Design review of the part built by this model. Coordinates are the model's own, in mm. A direction names the side the tool comes from. Coordinates: 2 decimals unless noted, no trailing zeros. Loops run counter-clockwise (first coordinate to the right, second up) from the corner with the lowest first, then second, coordinate; pieces in that order, holes last. Notation, with made-up numbers: (50, 74.25) - (92, 74.25) arc R19 ccw to (92, 92.25) - close; hole circle Ø2 at (6.5, 54). An arc over 180 degrees is marked (long way). Use one line per item in the form item = value. Start each with the question number.
(1) Clearance check with flat-ended pins moving along their axes: pin 1 Ø12 at (x, y) = (564, -11) entering from +Z; pin 2 Ø10 at (x, z) = (315.5, 11) entering from -Y; pin 3 Ø1.5 at (x, y) = (233.5, 1) entering from -Z; pin 4 Ø8 at (x, y) = (186.5, -3) entering from +Z. State where each tip first meets the part, or that it passes through.
(2) For L1, parallel to Z at x = 85, y = -23.5; L2, parallel to X at y = -25.5, z = 33.5; L3, parallel to Z at x = 700, y = 4, list the stretches that pass through material, from the lowest coordinate up.
(3) Add section B-B (x = 85). State the section outline as (y, z) points, plus the area to 3 significant figures.
(4) Add section C-C (z = -53). State the section outline as (x, y) points, plus the area to 3 significant figures.
(5) Tool access review of faces 1 (the face through (235.18, -9.86, 30.56)), 2 (the face through (396, -5, 1)), 3 (the face through (189.012, -16.504, -30.269)): name each direction out of +Z, -Z, +X, -X, +Y, -Y from which nothing blocks a thin tool from reaching the whole face with its end or side.
(6) The part is to be moulded in two halves that separate along X. For faces 4 (the face through (439.49, -3.5, -21.13)), 5 (the face through (685, -32.5, -17)), 6 (the face through (54.399, -9.86, -63.033)), say which applies: pulls with the +X half, pulls with the -X half, needs draft (parallel to the pull), parting line crosses it, or undercut.
(7) Add section A-A (y = 6). State the section outline as (x, z) points, plus the area to 3 significant figures.
```python
from build123d import *

# Parameters (mm, degrees)
F0_R          = 29
F1_DEPTH      = 20
F3_DEPTH      = 5
F5_DEPTH      = 5
F6_R          = 4.99999
F7_R          = 4.99999
F8_R          = 29
F8_R_2        = 22.5
F8_R_3        = 24
F9_DEPTH      = 12.5
F9_DEPTH_BACK = 32.5


# Not quite as in the source:
# - a fillet or chamfer is up to 0.001 mm smaller than in the source, because OpenCascade refuses the exact size


with BuildPart() as f1:
    # F0 (on Front) → F1 (new body)
    with BuildSketch(Plane.XZ):
        with BuildLine():
            Line((228.5028561992, 32.1062064806), (97.7975828549, 74.4774856478))
            ThreePointArc((97.7975828549, 74.4774856478), (54.8450921386, 63.5119541924), (46.3006134969, 20.0130895684))
            ThreePointArc((46.3006134969, 20.0130895684), (48.3193625322, 12.9155090118), (49, 5.5678746945))
            Line((49, 5.5678746945), (49, -5.5678746945))
            ThreePointArc((49, -5.5678746945), (48.3193625322, -12.9155090118), (46.3006134969, -20.0130895684))
            ThreePointArc((46.3006134969, -20.0130895684), (54.8450921386, -63.5119541924), (97.7975828549, -74.4774856478))
            Line((97.7975828549, -74.4774856478), (228.5028561992, -32.1062064806))
            ThreePointArc((228.5028561992, -32.1062064806), (235.0832865864, -30.5729005697), (241.8279137151, -30.1690491218))
            Line((241.8279137151, -30.1690491218), (698.9728356822, -41.4872864076))
            ThreePointArc((698.9728356822, -41.4872864076), (741.5, 0), (698.9728356822, 41.4872864076))
            Line((698.9728356822, 41.4872864076), (241.8279137151, 30.1690491218))
            ThreePointArc((241.8279137151, 30.1690491218), (235.0832865864, 30.5729005697), (228.5028561992, 32.1062064806))
        make_face()
        with Locations((85, -35)):
            Circle(F0_R, mode=Mode.SUBTRACT)
        with Locations((85, 35)):
            Circle(F0_R, mode=Mode.SUBTRACT)
        with Locations((700, 0)):
            Circle(F0_R, mode=Mode.SUBTRACT)
    extrude(amount=F1_DEPTH)

    # F2 (on face) → F3 (cut)
    with BuildSketch(Plane.XZ.offset(20)):
        with BuildLine():
            ThreePointArc((659.5520018106, -9.2849040098), (658.5, 0), (659.5520018106, 9.2849040098))
            ThreePointArc((659.5520018106, 9.2849040098), (656.5489690059, 22.1304501377), (644.5609792177, 27.6362981366))
            Line((644.5609792177, 27.6362981366), (240.0035775219, 17.6200506665))
            ThreePointArc((240.0035775219, 17.6200506665), (233.2589503932, 18.0239021144), (226.678520006, 19.5572080254))
            Line((226.678520006, 19.5572080254), (151.1675098096, 44.0359303551))
            ThreePointArc((151.1675098096, 44.0359303551), (133.238839262, 41.1870107565), (125, 25.010636067))
            Line((125, 25.010636067), (125, -25.010636067))
            ThreePointArc((125, -25.010636067), (133.238839262, -41.1870107565), (151.1675098096, -44.0359303551))
            Line((151.1675098096, -44.0359303551), (226.678520006, -19.5572080254))
            ThreePointArc((226.678520006, -19.5572080254), (233.2589503932, -18.0239021144), (240.0035775219, -17.6200506665))
            Line((240.0035775219, -17.6200506665), (644.5609792177, -27.6362981366))
            ThreePointArc((644.5609792177, -27.6362981366), (656.5489690059, -22.1304501377), (659.5520018106, -9.2849040098))
        make_face()
    extrude(amount=-F3_DEPTH, mode=Mode.SUBTRACT)

    # F4 (on face) → F5 (cut)
    with BuildSketch(Plane(origin=(0, 0, 0), x_dir=(-1, 0, 0), z_dir=(0, 1, 0))):
        with BuildLine():
            ThreePointArc((-659.5520018106, 9.2849040098), (-658.5, 0), (-659.5520018106, -9.2849040098))
            ThreePointArc((-659.5520018106, -9.2849040098), (-656.5489690059, -22.1304501377), (-644.5609792177, -27.6362981366))
            Line((-644.5609792177, -27.6362981366), (-240.0035775219, -17.6200506665))
            ThreePointArc((-240.0035775219, -17.6200506665), (-233.2589503932, -18.0239021144), (-226.678520006, -19.5572080254))
            Line((-226.678520006, -19.5572080254), (-151.1675098096, -44.0359303551))
            ThreePointArc((-151.1675098096, -44.0359303551), (-133.238839262, -41.1870107565), (-125, -25.010636067))
            Line((-125, -25.010636067), (-125, 25.010636067))
            ThreePointArc((-125, 25.010636067), (-133.238839262, 41.1870107565), (-151.1675098096, 44.0359303551))
            Line((-151.1675098096, 44.0359303551), (-226.678520006, 19.5572080254))
            ThreePointArc((-226.678520006, 19.5572080254), (-233.2589503932, 18.0239021144), (-240.0035775219, 17.6200506665))
            Line((-240.0035775219, 17.6200506665), (-644.5609792177, 27.6362981366))
            ThreePointArc((-644.5609792177, 27.6362981366), (-656.5489690059, 22.1304501377), (-659.5520018106, 9.2849040098))
        make_face()
    extrude(amount=-F5_DEPTH, mode=Mode.SUBTRACT)

    # F6 (radius 5 in the source; OpenCascade refuses exactly that, so slightly less here)
    f6_edges = [f1.edges().sort_by_distance(p)[0] for p in [
        (442.282278, -15, 22.628174),
    ]]
    fillet(f6_edges, radius=F6_R)

    # F7 (radius 5 in the source; OpenCascade refuses exactly that, so slightly less here)
    f7_edges = [f1.edges().sort_by_distance(p)[0] for p in [
        (442.282278, -5, 22.628174),
    ]]
    fillet(f7_edges, radius=F7_R)

    # F8 (on face) → F9 (join, two sides)
    with BuildSketch(Plane(origin=(0, 0, 0), x_dir=(-1, 0, 0), z_dir=(0, 1, 0))) as f9_sk:
        with Locations((-700, 0)):
            Circle(F8_R)
        with Locations((-700, 0)):
            Circle(F8_R_2, mode=Mode.SUBTRACT)
        with Locations((-85, 35)):
            Circle(F8_R)
        with Locations((-85, 35)):
            Circle(F8_R_3, mode=Mode.SUBTRACT)
        with Locations((-85, -35)):
            Circle(F8_R)
        with Locations((-85, -35)):
            Circle(F8_R_3, mode=Mode.SUBTRACT)
    extrude(amount=F9_DEPTH)
    extrude(f9_sk.sketch, amount=-F9_DEPTH_BACK)


solid = f1.part
```
Computed values:
q1.pin_1 = 38.29
q1.pin_2 = -15.23
q1.pin_3 = through
q1.pin_4 = 47.02
q2.L1 = -64 to -59, -11 to -6, 6 to 11, 59 to 64
q2.L2 = 56.04 to 61.05, 108.95 to 113.96
q2.L3 = -29 to -22.5, 22.5 to 29
q3.outline = (-32.5, -64) - (-20, -64) - (-20, -76.5) - (0, -76.5) - (0, -64) - (12.5, -64) - (12.5, -59) - (-32.5, -59) - close; (-32.5, -11) - (12.5, -11) - (12.5, -6) - (0, -6) - (0, 6) - (12.5, 6) - (12.5, 11) - (-32.5, 11) - (-32.5, 6) - (-20, 6) - (-20, -6) - (-32.5, -6) - close; (-32.5, 59) - (12.5, 59) - (12.5, 64) - (0, 64) - (0, 76.5) - (-20, 76.5) - (-20, 64) - (-32.5, 64) - close
q3.area = 1,640 mm^2
q4.outline = (47.61, -20) - (62.26, -20) - (62.26, -32.5) - (69.13, -32.5) - (69.13, 12.5) - (62.26, 12.5) - (62.26, 0) - (47.61, 0) - close; (100.87, -32.5) - (107.74, -32.5) - (107.74, -20) - (164.05, -20) - (164.05, 0) - (107.74, 0) - (107.74, 12.5) - (100.87, 12.5) - close
q4.area = 2,040 mm^2
q5.face_1 = +Z, +Y, -Y
q5.face_2 = +Y
q5.face_3 = -Y
q6.face_4 = undercut
q6.face_5 = needs draft
q6.face_6 = parting line crosses it
q7.outline = circle Ø58 at (85, -35); circle Ø58 at (85, 35); circle Ø58 at (700, 0); hole circle Ø48 at (85, -35); hole circle Ø48 at (85, 35); hole circle Ø45 at (700, 0)
q7.area = 2,720 mm^2
